Source: three-view drawing plus pictorial views. Frame: mm from the lowest corner of the part. A direction names the side the tool comes from. Give positions to 0.01 mm unless a question says otherwise; leave off trailing zeros. Order: outer loops, then holes, each group sorted by start corner. A loop starts at its lowest first (then second) coordinate and runs counter-clockwise, first axis right, second up. Notation, with made-up numbers: (-32, 19.25) -> (-1, 19.25) arc R32 cw to (-1, 49.25) -> close; hole circle Ø8 at (26, -10). An arc over 180 degrees is marked (long way). Write item = value, one per line.
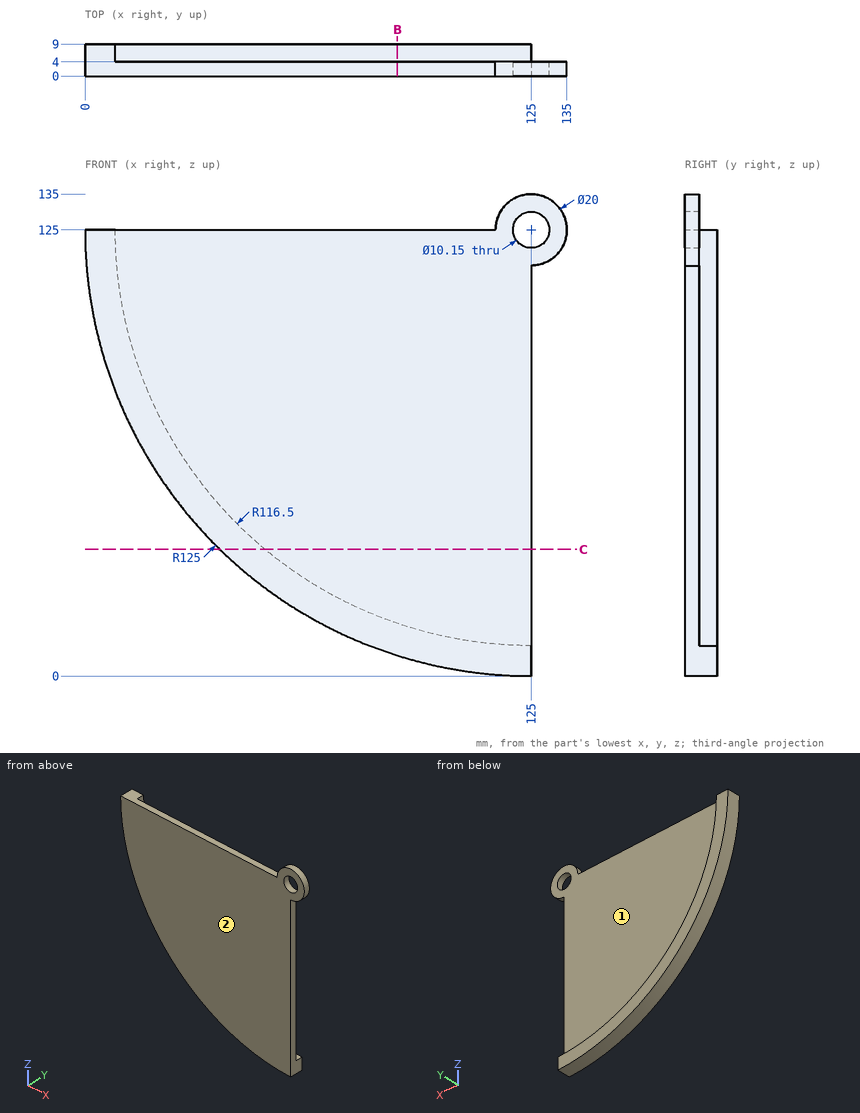
1) Line query: line 1 (Y direction, x = 73, z = 99.5); line 2 (X direction, y = 1, z = 92.5); line 3 (Z direction, x = 107, y = 6). Output: solid intervals per line, ascending. Write a range as from..to.
Check sheet entries:
line_1 = 0..4
line_2 = 4.3..125
line_3 = 1.3..9.9
2) Reachability of the marked faces 1 and 2 from +Z, -Z, +X, -X, +Y, -Y: full face, straight path, thin tool, end or side. Return the list, or none.
Check sheet entries:
face_1 = +Z, +X, +Y
face_2 = +Z, -Z, +X, -X, -Y
3) Section query C-C (z = 35.5). Output: boundary loops of the cut face in (x, y).
Check sheet entries:
outline = (37.74, 0) -> (125, 0) -> (125, 4) -> (50.42, 4) -> (50.42, 9) -> (37.74, 9) -> close
4) Section query B-B (x = 87.5). Output: boundary loops of the cut face in (y, z).
Check sheet entries:
outline = (0, 5.76) -> (9, 5.76) -> (9, 14.7) -> (4, 14.7) -> (4, 125) -> (0, 125) -> close
5) First-contact query: P1, Ø8, axis at x = 94.5, z = 75.5, coming from the +Y side; P2, Ø1, axis at x = 62.5, y = 7.5, coming from the -Z side; P3, Ø5, axis at x = 26, y = 5, coming from the -Z side. Flat tips, straight axial feed; report the tip coordinate or a pass-through.
Check sheet entries:
P1 = 4
P2 = 16.46
P3 = 45.55
